Verification items for the finished model (mm, model axes). A direction names the side the tool comes from. Round coordinates to 2 decimals unless told otherwise and drop trailing zeros. Write each loop counter-clockwise with the first axis right and the second up, starting at its lowest first coordinate (ties: lowest second). Pieces come first, ordered by that corner, then holes. Notation, with made-up numbers: (-38, -8) - (1, -8) arc R29 ccw to (1, 23) - close; hole circle Ø7 at (74.25, 36). An arc over 180 degrees is marked (long way). Answer as a JSON object with one key per item and string values.
```python
from build123d import *

# Parameters (mm, degrees)
CUT_EXTRUDE1_DEPTH = 2.159
CUT_EXTRUDE1_DRAFT = -5


with BuildPart() as part:
    # Sketch1 → Revolve1 (revolve)
    with BuildSketch(Plane.XY, mode=Mode.PRIVATE) as revolve1_sk:
        Polygon((1.4224, 0), (3.2385, 2.089184064), (0, 2.089184064), (0, 0), (0, -7.435815936), (1.4224, -7.435815936), align=None)
    revolve(revolve1_sk.sketch.rotate(Axis((0, 0, 0), (0, -1, 0)), 180), axis=Axis((0, 0, 0), (0, -1, 0)))


with BuildPart() as cut_extrude1_tool:
    # Sketch2 → Cut-Extrude1 (with draft: the straight prism first)
    with BuildSketch(Plane(origin=(0, 2.089184064, 0), x_dir=(1, 0, 0), z_dir=(0, 1, 0))):
        Polygon((-0.381, 1.524), (-0.381, 0.381), (-1.524, 0.381), (-1.524, -0.381), (-0.381, -0.381), (-0.381, -1.524), (0.381, -1.524), (0.381, -0.381), (1.524, -0.381), (1.524, 0.381), (0.381, 0.381), (0.381, 1.524), align=None)
    extrude(amount=-CUT_EXTRUDE1_DEPTH)
    # Cut-Extrude1: the draft: its side faces are tilted about the plane it starts from
    cut_extrude1_sides = [cut_extrude1_tool.faces().sort_by_distance(p)[0] for p in [
        (-0.381, 1.009684064, -0.9525),
        (-0.9525, 1.009684064, -0.381),
        (-1.524, 1.009684064, 0),
        (-0.9525, 1.009684064, 0.381),
        (-0.381, 1.009684064, 0.9525),
        (0, 1.009684064, 1.524),
        (0.381, 1.009684064, 0.9525),
        (0.9525, 1.009684064, 0.381),
        (1.524, 1.009684064, 0),
        (0.9525, 1.009684064, -0.381),
        (0.381, 1.009684064, -0.9525),
        (0, 1.009684064, -1.524),
    ]]
    draft(cut_extrude1_sides, Plane(origin=(0, 2.089184064, 0), x_dir=(1, 0, 0), z_dir=(0, 1, 0)), CUT_EXTRUDE1_DRAFT)


with BuildPart() as part_1:
    add(part.part)

    # Cut-Extrude1: cut by cut_extrude1_tool
    add(cut_extrude1_tool.part, mode=Mode.SUBTRACT)


solid = part_1.part
```
1. Mould release check, pull along Z, two halves, no side actions. Record for faces 1 (the face through (-0.66, -3.67, 1.26)), 2 (the face through (-1, 2.089, 1)), 3 (the face through (0.867, 1.025, -0.288)): released by +Z, released by -Z, zero draft, split by the parting line, or undercut.
Completed:
{"face 1": "split by the parting line", "face 2": "zero draft", "face 3": "undercut"}
2. Cross-section at B-B (z = 0). Record the boundary of the cut face in (x, y), plus the area to 3 significant figures.
Completed:
{"outline": "(-3.24, 2.09) - (-1.42, 0) - (-1.42, -7.44) - (1.42, -7.44) - (1.42, 0) - (3.24, 2.09) - (1.52, 2.09) - (1.34, -0.07) - (-1.34, -0.07) - (-1.52, 2.09) - close", "area": "24.7 mm^2"}
3. Cross-section at A-A (y = 0.25). Record the boundary of the cut face in (x, z).
Completed:
{"outline": "circle Ø3.28 at (0, 0); hole (-1.36, -0.22) - (-0.22, -0.22) - (-0.22, -1.36) - (0.22, -1.36) - (0.22, -0.22) - (1.36, -0.22) - (1.36, 0.22) - (0.22, 0.22) - (0.22, 1.36) - (-0.22, 1.36) - (-0.22, 0.22) - (-1.36, 0.22) - close"}
4. Go/stop test with flat-tipped pins: pin 1 (2 mm diameter, centred on y = 0.5, z = 1, fed in from +X); pin 2 (1.5 mm diameter, centred on y = -5, z = 1.5, fed in from +X); pin 3 (1 mm diameter, centred on y = -4.5, z = 0, fed in from +X). Record where each tip stops, or that it passes through.
Completed:
{"pin 1": "stops at x = 2.59", "pin 2": "stops at x = 1.21", "pin 3": "stops at x = 1.42"}
5. Cross-section at C-C (x = 0). Record the boundary of the cut face in (y, z).
Completed:
{"outline": "(-7.44, -1.42) - (0, -1.42) - (2.09, -3.24) - (2.09, -1.52) - (-0.07, -1.34) - (-0.07, 1.34) - (2.09, 1.52) - (2.09, 3.24) - (0, 1.42) - (-7.44, 1.42) - close"}
6. Access from +Z, -Z, +X, -X, +Y, -Y to the whole of each face (thin tool, end or side, straight path). Record for faces 4 (the face through (0, -0.07, 0)), 5 (the face through (0, -7.436, 0)).
Completed:
{"face 4": "+Y", "face 5": "+Z, -Z, +X, -X, -Y"}
7. Material ranges on probe 1 along Y at (x, z) = (0, -0.75); probe 2 along X at (y, z) = (1, 0.75); probe 3 along X at (y, z) = (-6, 0.5), recorded low to high. Write a range as from..to.
Completed:
{"probe 1": "y = -7.44..-0.07", "probe 2": "x = -2.17..-0.29, 0.29..2.17", "probe 3": "x = -1.33..1.33"}
8. Cross-section at D-D (y = -2). Record the boundary of the cut face in (x, z).
Completed:
{"outline": "circle Ø2.84 at (0, 0)"}
